Autodesk Fusion 360 part; units mm, degrees
sketch "Sketch1" plane through (0, 0, 0) normal (1, 0, 0) x (0, 0, -1)
  circle A0 centre (0, 0) radius 40
  line L0 (-2.9, 1.75) -> (2.9, 1.75)
  line L1 (2.9, 1.75) -> (2.9, -1.75)
  line L2 (2.9, -1.75) -> (-2.9, -1.75)
  line L3 (-2.9, -1.75) -> (-2.9, 1.75)
  line L4 (-2.9, 1.75) -> (2.9, -1.75) construction
  line L5 (2.9, 1.75) -> (-2.9, -1.75) construction
  dimension "d1" = 80
  dimension "d2" = 5.8
  dimension "d3" = 3.5
sketch "Sketch2" plane through (0, 0, 0) normal (0, 1, 0) x (1, 0, 0)
  line L0 (16.6, 6) -> (-16.6, 6)
  line L1 (-16.6, 6) -> (-16.6, -6)
  line L2 (-16.6, -6) -> (16.6, -6)
  line L3 (16.6, -6) -> (16.6, 6)
  line L4 (16.6, 6) -> (-16.6, -6) construction
  line L5 (-16.6, 6) -> (16.6, -6) construction
  dimension "d6" = 33.2
  dimension "d7" = 12
extrude "Extrude2" add sketch "Sketch2" along normal blind 10 makes body 1
sketch "Sketch3" plane through (16.6, 0, 0) normal (1, 0, 0) x (0, 0, -1)
  line L0 (-6, 0) -> (6, 0)
  line L1 (6, 0) -> (6, 10)
  line L2 (6, 10) -> (-6, 10)
  line L3 (-6, 10) -> (-6, 0)
  circle A0 centre (-0.0016, 5.0186) radius 1.5
  line L4 (-1.2598, 5.8353) -> (1.2566, 5.8353)
  dimension "d10" = 3
extrude "Extrude3" add sketch "Sketch3" along normal blind 15 contours A0 L4 picked at (-0.2512, 6.075) bodies 1
sketch "Sketch4" plane through (0, 0, 0) normal (1, 0, 0) x (0, 0, -1)
  circle A0 centre (0, 0) radius 30
  dimension "d13" = 60
extrude "Extrude4" add sketch "Sketch4" along normal blind 8 separate body makes body 2
sketch "Sketch5" plane through (0, 0, 0) normal (-1, 0, 0) x (0, 0, 1)
  circle A0 centre (0, 0) radius 30
  circle A1 centre (0, 0) radius 1.5
  line L0 (-1.26, 0.8139) -> (1.26, 0.8139)
  dimension "d20" = 3
  dimension "d21" = 2.52
extrude "Extrude5" cut sketch "Sketch5" against normal blind 14 contours A1 L0 picked at (0.3772, 0.8708) bodies 2
copy_body "Body->Comp1" bodies 2 removing the originals makes body 3 in component "Component"
component "Component" placed x (1, 0, 0) y (0, 1, 0) z (0, 0, 1) at (0, 0, 0)
hidden bodies 3
Work out the finished part from the listing and answer in its coordinate system (mm). A direction names the side the tool comes from. Round coordinates to 2 decimals unless told otherwise and drop trailing zeros. Loops run counter-clockwise (first coordinate to the right, second up) from the corner with the lowest first, then second, coordinate; pieces in that order, holes last. Notation, with made-up numbers: M 54.5,-36.75 L 105.5,-36.75 A29 ccw 105.5,-14.75 Z; hole C 74.25,83.25 d7. An arc over 180 degrees is marked long. One line per question, with ' | ' between items. Start each with the question number.
(1) A cutting plane is placed at C-C on z = 4. Write down the section's boundary in (x, y), plus the area to 3 significant figures.
(2) A cutting plane is placed at B-B on y = 7.25. Write down the section's boundary in (x, z).
(3) A tool of negligible diameter and unlimited length cuts with its end or side. For faces 1 (the face through (24, 5.835, 0)), 2 (the face through (0, 0, 0)), 3 (the face through (24, 6.52, 0.02)), from which of +Z, -Z, +X, -X, +Y, -Y can it reach the whole face along a straight path? Write none if from no direction.
(4) Flat-ended cylindrical pins translate along their axes: pin 1 Ø4 at (y, z) = (3.5, -1.5) entering from +X; pin 2 Ø2 at (x, z) = (22, 0) entering from -Y. Find the tip coordinate at first contact, or state that the pin passes through.
(5) Find the intervals of material crossed by line 1 (X direction, y = 6, z = -5), in increasing order.
(6) A cutting plane is placed at A-A on z = 0.25. Write down the section's boundary in (x, y), plus the area to 3 significant figures.
Geometry check:
1) outline: M -16.6,0 L 16.6,0 L 16.6,10 L -16.6,10 Z | area: 332 mm²
2) outline: M -16.6,-6 L 16.6,-6 L 16.6,6 L -16.6,6 Z
3) face 1: +Z, -Z, +X, -Y | face 2: +Z, -Z, +X, -X, -Y | face 3: +X, +Y
4) pin 1: stops at x = 16.6 | pin 2: stops at y = 5.84
5) line 1: x = -16.6 to 16.6
6) outline: M -16.6,0 L 16.6,0 L 16.6,5.84 L 31.6,5.84 L 31.6,6.5 L 16.6,6.5 L 16.6,10 L -16.6,10 Z | area: 342 mm²
